```python
from build123d import *

# Parameters (mm, degrees)
F0_R     = 16.475764
F1_DEPTH = 50.8
F0_W     = 141.873404
F0_H     = 107.963092
F2_DEPTH = 25.4
F4_DEPTH = 107.964093


with BuildPart() as f1:
    # F0 (on Top) → F1 (new body)
    with BuildSketch(Plane.XY):
        Circle(F0_R)
    extrude(amount=F1_DEPTH)

    # F0 (on Top) → F2 (join)
    with BuildSketch(Plane.XY):
        Rectangle(F0_W, F0_H)
        Circle(F0_R, mode=Mode.SUBTRACT)
    extrude(amount=F2_DEPTH)

    # F3 (on face) → F4 (cut, through all)
    with BuildSketch(Plane.XZ.offset(53.981546)):
        Polygon((16.475764, 50.8), (-16.475764, 50.8), (16.475764, 38.1), align=None)
    extrude(amount=-F4_DEPTH, mode=Mode.SUBTRACT)


solid = f1.part
```
The model under review builds one solid part; all positions refer to its coordinate system, in mm. A direction names the side the tool comes from. Coordinates: 2 decimals unless noted, no trailing zeros. Order: outer loops, then holes, each group sorted by start corner. A loop starts at its lowest first (then second) coordinate and runs counter-clockwise, first axis right, second up. Notation, with made-up numbers: M 88.5,-28 L 101.5,-28 A11 ccw 101.5,-17 Z; hole C 48.5,-39 d6. An arc over 180 degrees is marked long. One line per question, with ' | ' between items.
(1) Add section D-D, the plane x = -57. Write out the cut boundary in (y, z), then the cut area to 3 significant figures.
Geometry results:
outline: M -53.98,0 L 53.98,0 L 53.98,25.4 L -53.98,25.4 Z | area: 2,740 mm²
(2) Add section C-C, the plane z = 47. Write out the cut boundary in (x, y).
Geometry results:
outline: M -6.62,-15.09 L -6.62,15.09 A16.48 ccw Z
(3) For probe 1 along Z at (x, y) = (0.5, 40); probe 2 along Z at (x, y) = (1, 13.5); probe 3 along Y at (x, z) = (13, 32.5), list the stretches that pass through material, from the lowest coordinate up. Write a range as from..to.
Geometry results:
probe 1: z = 0..25.4 | probe 2: z = 0..44.06 | probe 3: y = -10.12..10.12
(4) Machinability: for faces 1 (the face through (-1, -53.982, 13)), 2 (the face through (-16.46, 0.72, 35.1)), which of the approach directions +Z, -Z, +X, -X, +Y, -Y give a long, thin tool a straight path to every point of the face, cutting with its end or side? Answer none if there is none.
Geometry results:
face 1: +Z, -Z, +X, -X, -Y | face 2: +Z
(5) Add section A-A, the plane y = 0. Write out the cut boundary in (x, z), then the cut area to 3 significant figures.
Geometry results:
outline: M -70.94,0 L 70.94,0 L 70.94,25.4 L 16.48,25.4 L 16.48,38.1 L -16.48,50.8 L -16.48,25.4 L -70.94,25.4 Z | area: 4,230 mm²
(6) Insertion check: pin 1 (8 mm diameter, centred on x = -21.5, z = 40.5, fed in from +Y); pin 2 (4 mm diameter, centred on x = -46.5, y = 13, fed in from +Z); pin 3 (1.5 mm diameter, centred on x = -0.5, z = 30, fed in from -Y); pin 4 (4 mm diameter, centred on x = -3, z = 42, fed in from +Y). Each pin has a flat end and moves straight along its axis. Give the tip position at first contact, or say it passes through.
Geometry results:
pin 1: passes through | pin 2: stops at z = 25.4 | pin 3: stops at y = -16.48 | pin 4: stops at y = 16.45
(7) Add section B-B, the plane x = 0. Write out the cut boundary in (y, z), then the cut area to 3 significant figures.
Geometry results:
outline: M -53.98,0 L 53.98,0 L 53.98,25.4 L 16.48,25.4 L 16.48,44.45 L -16.48,44.45 L -16.48,25.4 L -53.98,25.4 Z | area: 3,370 mm²
